Can you work these out from the model? Positions are in its coordinate system, mm. A direction names the side the tool comes from. Coordinates: 2 decimals unless noted, no trailing zeros. Order: outer loops, then holes, each group sorted by start corner. A loop starts at its lowest first (then second) coordinate and runs counter-clockwise, first axis right, second up. Notation, with made-up numbers: (81, 77.25) -> (85, 77.25) arc R9 cw to (85, 85.25) -> close; hole circle Ø10 at (36, 62). An arc over 180 degrees is marked (long way). Write item = value, one per line. Start each with the question number.
from build123d import *

# Parameters (mm, degrees)
F0_W     = 54
F0_H     = 82
F0_R     = 2.5
F0_R_2   = 8
F1_DEPTH = 10
F2_SIZE  = 3
F3_W     = 30
F3_H     = 82
F4_DEPTH = 2


with BuildPart() as f1:
    # F0 (on Top) → F1 (new body)
    with BuildSketch(Plane.XY):
        Rectangle(F0_W, F0_H)
        with Locations((-19, -33)):
            Circle(F0_R, mode=Mode.SUBTRACT)
        with Locations((0, -26)):
            Circle(F0_R_2, mode=Mode.SUBTRACT)
        with Locations((19, -33)):
            Circle(F0_R, mode=Mode.SUBTRACT)
        with Locations((-19, 0)):
            Circle(F0_R, mode=Mode.SUBTRACT)
        with Locations((-19, 33)):
            Circle(F0_R, mode=Mode.SUBTRACT)
        with Locations((19, 0)):
            Circle(F0_R, mode=Mode.SUBTRACT)
        with Locations((0, 26)):
            Circle(F0_R_2, mode=Mode.SUBTRACT)
        with Locations((19, 33)):
            Circle(F0_R, mode=Mode.SUBTRACT)
    extrude(amount=F1_DEPTH)

    # F2
    f2_edges = [f1.edges().sort_by_distance(p)[0] for p in [
        (27, -41, 5),
        (-27, -41, 5),
        (27, 41, 5),
        (-27, 41, 5),
    ]]
    chamfer(f2_edges, length=F2_SIZE)

    # F3 (on face) → F4 (cut)
    with BuildSketch(Plane.XY.offset(10)):
        Rectangle(F3_W, F3_H)
    extrude(amount=-F4_DEPTH, mode=Mode.SUBTRACT)


solid = f1.part
(1) Imagine slicing it at C-C (y = 26). Write out the boundary of the cut face in (x, z).
(2) Thinking about a two-plate mould opening in X: for faces 1 (the face through (-15, -1, 9)), 2 (the face through (-25, -40, 5)), 3 (the face through (26, -39, 5)), which applies, +X half, -X half, draft (parallel to the pull), parting line (faces both ways), or undercut?
(3) Imagine slicing it at A-A (x = 19). Write out the boundary of the cut face in (y, z).
(4) If I drill on L1, parallel to Y at x = 0, z = 4.75; L2, parallel to Y at x = -19, z = 6.75; L3, parallel to X at y = 31, z = 7.25 (3 decimals), over which ranges is the centre line in solid material (lowest first)? Write a range as from..to.
(5) For faces 4 (the face through (-27, -1, 5)), 5 (the face through (0, 1, 8)), which set-ups out of +Z, -Z, +X, -X, +Y, -Y let a thin tool reach every point of the face, with its end or its side?
(6) For P1, Ø6.5, axis at x = -19, y = 0, coming from the +Z side; P2, Ø8, axis at x = 7.5, y = 27, coming from the +Z side, each with a flat end and sliding along its axis, tell me the tip position at first contact or that it passes through.
(7) Imagine slicing it at D-D (x = 0). Write out the boundary of the cut face in (y, z).
(8) Imagine slicing it at B-B (z = 5.5). Count the separate pieces of the cut face and the enclosed holes in it, plus the area to 3 significant figures.
Result set:
q1.outline = (-27, 0) -> (-8, 0) -> (-8, 8) -> (-15, 8) -> (-15, 10) -> (-27, 10) -> close; (8, 0) -> (27, 0) -> (27, 10) -> (15, 10) -> (15, 8) -> (8, 8) -> close
q2.face_1 = undercut
q2.face_2 = -X half
q2.face_3 = +X half
q3.outline = (-41, 0) -> (-35.5, 0) -> (-35.5, 10) -> (-41, 10) -> close; (-30.5, 0) -> (-2.5, 0) -> (-2.5, 10) -> (-30.5, 10) -> close; (2.5, 0) -> (30.5, 0) -> (30.5, 10) -> (2.5, 10) -> close; (35.5, 0) -> (41, 0) -> (41, 10) -> (35.5, 10) -> close
q4.L1 = -41..-34, -18..18, 34..41
q4.L2 = -41..-35.5, -30.5..-2.5, 2.5..30.5, 35.5..41
q4.L3 = -27..-20.5, -17.5..-6.245, 6.245..17.5, 20.5..27
q5.face_4 = +Z, -Z, -X, +Y, -Y
q5.face_5 = +Z, +Y, -Y
q6.P1 = 10
q6.P2 = 8
q7.outline = (-41, 0) -> (-34, 0) -> (-34, 8) -> (-41, 8) -> close; (-18, 0) -> (18, 0) -> (18, 8) -> (-18, 8) -> close; (34, 0) -> (41, 0) -> (41, 8) -> (34, 8) -> close
q8.separate_pieces = 1
q8.enclosed_holes = 8
q8.area = 3,890 mm2
